from build123d import *

# Parameters (mm, degrees)
F0_R     = 107.7630734498
F0_R_2   = 12.7
F1_DEPTH = 6.35
F2_DEPTH = 12.7
F3_R     = 133.1630796194
F4_DEPTH = 3.175


with BuildPart() as f1:
    # F0 (on Top) → F1 (new body)
    with BuildSketch(Plane.XY):
        Circle(F0_R)
        Circle(F0_R_2, mode=Mode.SUBTRACT)
        Circle(F0_R_2)
    extrude(amount=F1_DEPTH)

    # F0 (on Top) → F2 (join)
    with BuildSketch(Plane.XY):
        Circle(F0_R_2)
    extrude(amount=-F2_DEPTH)

    # F3 (on face) → F4 (join)
    with BuildSketch(Plane(origin=(0, 0, -12.7), x_dir=(1, 0, 0), z_dir=(0, 0, -1))):
        Circle(F3_R)
        with BuildLine():
            ThreePointArc((6.35, 107.5758220947), (78.4129310629, 73.9208511955), (107.7630734498, 0))
            ThreePointArc((107.7630734498, 0), (78.4129310629, -73.9208511955), (6.35, -107.5758220947))
            Line((6.35, -107.5758220947), (6.35, -123.9275708795))
            Line((6.35, -123.9275708795), (-6.35, -123.9275708795))
            Line((-6.35, -123.9275708795), (-6.35, -107.5758220947))
            ThreePointArc((-6.35, -107.5758220947), (-107.7630734498, 0), (-6.35, 107.5758220947))
            Line((-6.35, 107.5758220947), (-6.35, 123.9275708795))
            Line((-6.35, 123.9275708795), (6.35, 123.9275708795))
            Line((6.35, 123.9275708795), (6.35, 107.5758220947))
        make_face(mode=Mode.SUBTRACT)
        with BuildLine():
            ThreePointArc((-6.35, -107.5758220947), (0, -107.7630734498), (6.35, -107.5758220947))
            Line((6.35, -107.5758220947), (6.35, -10.9985226281))
            ThreePointArc((6.35, -10.9985226281), (0, -12.7), (-6.35, -10.9985226281))
            Line((-6.35, -10.9985226281), (-6.35, -107.5758220947))
        make_face()
        with BuildLine():
            Line((6.35, 10.9985226281), (6.35, 107.5758220947))
            ThreePointArc((6.35, 107.5758220947), (0, 107.7630734498), (-6.35, 107.5758220947))
            Line((-6.35, 107.5758220947), (-6.35, 10.9985226281))
            ThreePointArc((-6.35, 10.9985226281), (0, 12.7), (6.35, 10.9985226281))
        make_face()
        with BuildLine():
            Line((6.35, -123.9275708795), (6.35, -107.5758220947))
            ThreePointArc((6.35, -107.5758220947), (0, -107.7630734498), (-6.35, -107.5758220947))
            Line((-6.35, -107.5758220947), (-6.35, -123.9275708795))
            Line((-6.35, -123.9275708795), (6.35, -123.9275708795))
        make_face()
        with BuildLine():
            ThreePointArc((-6.35, 107.5758220947), (0, 107.7630734498), (6.35, 107.5758220947))
            Line((6.35, 107.5758220947), (6.35, 123.9275708795))
            Line((6.35, 123.9275708795), (-6.35, 123.9275708795))
            Line((-6.35, 123.9275708795), (-6.35, 107.5758220947))
        make_face()
    extrude(amount=-F4_DEPTH)


solid = f1.part
Design review of the part built by this model. Coordinates are the model's own, in mm. A direction names the side the tool comes from. Round coordinates to 2 decimals unless told otherwise and drop trailing zeros. Loops run counter-clockwise (first coordinate to the right, second up) from the corner with the lowest first, then second, coordinate; pieces in that order, holes last. Notation, with made-up numbers: (61.5, 46) - (72.5, 46) arc R24 ccw to (72.5, 72) - close; hole circle Ø8 at (8.5, 84.25). An arc over 180 degrees is marked (long way). One line per question, with ' | ' between items.
1. We need section A-A, the plane y = 81. State the section outline as (x, z) points (3 decimals).
Results are:
outline: (-105.695, -12.7) - (-71.077, -12.7) - (-71.077, -9.525) - (-105.695, -9.525) - close; (-71.077, 0) - (71.077, 0) - (71.077, 6.35) - (-71.077, 6.35) - close; (-6.35, -12.7) - (6.35, -12.7) - (6.35, -9.525) - (-6.35, -9.525) - close; (71.077, -12.7) - (105.695, -12.7) - (105.695, -9.525) - (71.077, -9.525) - close
2. We need section C-C, the plane x = 0. State the section outline as (y, z) points (3 decimals).
Results are:
outline: (-133.163, -12.7) - (133.163, -12.7) - (133.163, -9.525) - (12.7, -9.525) - (12.7, 0) - (107.763, 0) - (107.763, 6.35) - (-107.763, 6.35) - (-107.763, 0) - (-12.7, 0) - (-12.7, -9.525) - (-133.163, -9.525) - close
3. We need section D-D, the plane y = -66. State the section outline as (x, z) points (3 decimals), and give its area (3 significant figures).
Results are:
outline: (-115.656, -12.7) - (-85.187, -12.7) - (-85.187, -9.525) - (-115.656, -9.525) - close; (-85.187, 0) - (85.187, 0) - (85.187, 6.35) - (-85.187, 6.35) - close; (-6.35, -12.7) - (6.35, -12.7) - (6.35, -9.525) - (-6.35, -9.525) - close; (85.187, -12.7) - (115.656, -12.7) - (115.656, -9.525) - (85.187, -9.525) - close | area: 1,320 mm²
4. Clearance check with flat-ended pins moving along their axes: P1, Ø1.6, axis at y = -46.5, z = -10.5, coming from the -X side; P2, Ø2.5, axis at y = 66.5, z = -11.5, coming from the -X side; P3, Ø3.5, axis at y = 38, z = -11, coming from the +X side. State where each tip first meets the part, or that it passes through.
Results are:
P1: stops at x = -125.08 | P2: stops at x = -116.08 | P3: stops at x = 128.13
5. We need section B-B, the plane x = -90. State the section outline as (y, z) points (3 decimals), and give its area (4 significant figures).
Results are:
outline: (-98.145, -12.7) - (-59.27, -12.7) - (-59.27, -9.525) - (-98.145, -9.525) - close; (-59.27, 0) - (59.27, 0) - (59.27, 6.35) - (-59.27, 6.35) - close; (59.27, -12.7) - (98.145, -12.7) - (98.145, -9.525) - (59.27, -9.525) - close | area: 1,000 mm²
6. For L1, parallel to X at y = 84, z = -10.5; L2, parallel to Z at x = 25.5, y = -52.5; L3, parallel to Z at x = -24, y = -113 (3 decimals), list the stretches that pass through material, from the lowest coordinate up. Write a range as [from, to].
Results are:
L1: x = [-103.33, -67.5], [-6.35, 6.35], [67.5, 103.33] | L2: z = [0, 6.35] | L3: z = [-12.7, -9.525]
7. Draft analysis for pull direction X (two halves, no side actions). For faces 1 (the face through (-107.74, 2.28, -11.13)), 2 (the face through (-107.66, 4.74, 3.13)), 3 (the face through (-2, -22, 0)), state which applies: released by +X, released by -X, zero draft, split by the parting line, or undercut.
Results are:
face 1: undercut | face 2: split by the parting line | face 3: zero draft
8. For faces 4 (the face through (-1.653, 12.592, -6.261)), 5 (the face through (-2, 2, 6.35)), list the 3-axis set-ups (+Z, -Z, +X, -X, +Y, -Y) from which the entire face can be reached by the end or side of a thin tool; tool diameter is ignored.
Results are:
face 4: none | face 5: +Z, +X, -X, +Y, -Y
